```python
from build123d import *

# Parameters (mm, degrees)
SKETCH1_R           = 20
BOSS_EXTRUDE1_DEPTH = 10
SKETCH2_R           = 16
CUT_EXTRUDE1_DEPTH  = 7
SKETCH3_R           = 1.55
CUT_EXTRUDE2_DEPTH  = 4
CHAMFER1_SIZE       = 2


with BuildPart() as part:
    # Sketch1 → Boss-Extrude1 (new body)
    with BuildSketch(Plane.XY):
        Circle(SKETCH1_R)
    extrude(amount=BOSS_EXTRUDE1_DEPTH)

    # Sketch2 → Cut-Extrude1 (cut)
    with BuildSketch(Plane.XY.offset(10)):
        Circle(SKETCH2_R)
    extrude(amount=-CUT_EXTRUDE1_DEPTH, mode=Mode.SUBTRACT)

    # Sketch3 → Cut-Extrude2 (cut, through all)
    with BuildSketch(Plane.XY.offset(3)):
        with Locations((0, -5)):
            Circle(SKETCH3_R)
        with Locations((0, 5)):
            Circle(SKETCH3_R)
    extrude(amount=-CUT_EXTRUDE2_DEPTH, mode=Mode.SUBTRACT)

    # Chamfer1
    chamfer1_edges = [part.edges().sort_by_distance(p)[0] for p in [
        (-1.55, -5, 3),
        (-1.55, 5, 3),
    ]]
    chamfer(chamfer1_edges, length=CHAMFER1_SIZE)


solid = part.part
```
Read the model definition and answer for the solid it produces. Units are mm, in the model's axes. A direction names the side the tool comes from. Round coordinates to 2 decimals unless told otherwise and drop trailing zeros. Write each loop counter-clockwise with the first axis right and the second up, starting at its lowest first coordinate (ties: lowest second). Pieces come first, ordered by that corner, then holes. Notation, with made-up numbers: (53.25, -18.75) -> (70.25, -18.75) arc R25 cw to (70.25, -5.75) -> close; hole circle Ø7 at (-23, 16). An arc over 180 degrees is marked (long way). Answer in a Markdown table with one row per item. Add a question column.
1) Find section A-A, the plane x = 0. Determine the outline of the cut face in (y, z), and give its area (3 significant figures).
2) Find section B-B, the plane y = -5. Determine the outline of the cut face in (x, z), and give its area (3 significant figures).
3) Given P1, Ø1, axis at x = 1, z = 2.5, coming from the -Y side; P2, Ø3, axis at y = -2.5, z = 4, coming from the +X side (3 decimals); P3, Ø4, axis at x = 13, z = 7.5, coming from the -Y side, each flat-ended and moving along its own axis, determine where each tip first touches the part or whether it passes through.
4) Find section D-D, the plane y = 0. Determine the outline of the cut face in (x, z), and give its area (3 significant figures).
5) Which of the six approach directions +Z, -Z, +X, -X, +Y, -Y give full straight-line access (tool end or side, diameter ignored) to faces 5 (the face through (-3.47, -15.62, 6.55)), 6 (the face through (0, 0, 0))?
6) Consider line 1 (Y direction, x = 0, z = 0.45); line 2 (Z direction, x = -1, y = 1.5); line 3 (Y direction, x = -3, z = 4). Determine where each line is inside the solid, lowest interval first.
7) Determine the mould class of faces 1 (the face through (-4.336, -19.524, 4.93)), 2 (the face through (0, 0, 3)), 3 (the face through (1.547, 4.358, 1.125)), 4 (the face through (-8.98, 13.43, 10)) for opening direction Y: pulls with the +Y half, pulls with the -Y half, needs draft (parallel to the pull), parting line crosses it, or undercut.
8) Find section C-C, the plane z = 2.5. Determine the outline of the cut face in (x, y), and give its area (3 significant figures).
Findings below:
| question | item | result |
|---|---|---|
| 1 | outline | (-20, 0) -> (-6.55, 0) -> (-6.55, 1) -> (-8.55, 3) -> (-16, 3) -> (-16, 10) -> (-20, 10) -> close; (-3.45, 0) -> (3.45, 0) -> (3.45, 1) -> (1.45, 3) -> (-1.45, 3) -> (-3.45, 1) -> close; (6.55, 0) -> (20, 0) -> (20, 10) -> (16, 10) -> (16, 3) -> (8.55, 3) -> (6.55, 1) -> close |
| 1 | area | 149 mm² |
| 2 | outline | (-19.36, 0) -> (-1.55, 0) -> (-1.55, 1) -> (-3.55, 3) -> (-15.2, 3) -> (-15.2, 10) -> (-19.36, 10) -> close; (1.55, 0) -> (19.36, 0) -> (19.36, 10) -> (15.2, 10) -> (15.2, 3) -> (3.55, 3) -> (1.55, 1) -> close |
| 2 | area | 161 mm² |
| 3 | P1 | y = -19.99 |
| 3 | P2 | x = 19.975 |
| 3 | P3 | y = -16.7 |
| 4 | outline | (-20, 0) -> (20, 0) -> (20, 10) -> (16, 10) -> (16, 3) -> (-16, 3) -> (-16, 10) -> (-20, 10) -> close |
| 4 | area | 176 mm² |
| 5 | face 5 | +Z |
| 5 | face 6 | -Z, +X, -X, +Y, -Y |
| 6 | line 1 | -20 to -6.55, -3.45 to 3.45, 6.55 to 20 |
| 6 | line 2 | 0 to 3 |
| 6 | line 3 | -19.77 to -15.72, 15.72 to 19.77 |
| 7 | face 1 | parting line crosses it |
| 7 | face 2 | undercut |
| 7 | face 3 | undercut |
| 7 | face 4 | needs draft |
| 8 | outline | circle Ø40 at (0, 0); hole circle Ø6.1 at (0, -5); hole circle Ø6.1 at (0, 5) |
| 8 | area | 1,200 mm² |
